Source: CAD feature listing. Evaluate the final solid. Frame: model axes, mm. A direction names the side the tool comes from. Give positions to 0.01 mm unless a question says otherwise; leave off trailing zeros. Order: outer loops, then holes, each group sorted by start corner. A loop starts at its lowest first (then second) coordinate and runs counter-clockwise, first axis right, second up.
from build123d import *

# Parameters (mm, degrees)
SKETCH1_R           = 11.5
BOSS_EXTRUDE1_DEPTH = 19
SKETCH2_R           = 0.6
BOSS_EXTRUDE4_DEPTH = 19
SKETCH3_R           = 3
BOSS_EXTRUDE5_DEPTH = 8.5
SKETCH4_R           = 1
CUT_EXTRUDE1_DEPTH  = 8.5


with BuildPart() as part:
    # Sketch1 → Boss-Extrude1 (new body)
    with BuildSketch(Plane.XY):
        Circle(SKETCH1_R)
    extrude(amount=BOSS_EXTRUDE1_DEPTH)

    # Sketch2 → Boss-Extrude4 (add)
    with BuildSketch(Plane(origin=(0, 0, 0), x_dir=(1, 0, 0), z_dir=(0, 1, 0))):
        with Locations((-2.2, -18.2)):
            Circle(SKETCH2_R)
        with Locations((-1.1, -18.2)):
            Circle(SKETCH2_R)
        with Locations((0, -18.2)):
            Circle(SKETCH2_R)
        with Locations((1.1, -18.2)):
            Circle(SKETCH2_R)
        with Locations((2.2, -18.2)):
            Circle(SKETCH2_R)
    extrude(amount=BOSS_EXTRUDE4_DEPTH)

    # Sketch3 → Boss-Extrude5 (add)
    with BuildSketch(Plane(origin=(0, 0, 0), x_dir=(-1, 0, 0), z_dir=(0, 0, -1))):
        Circle(SKETCH3_R)
    extrude(amount=BOSS_EXTRUDE5_DEPTH)

    # Sketch4 → Cut-Extrude1 (cut)
    with BuildSketch(Plane(origin=(0, 0, 0), x_dir=(-1, 0, 0), z_dir=(0, 0, -1))):
        with Locations((0, -8.5)):
            Circle(SKETCH4_R)
        with Locations((0, 8.5)):
            Circle(SKETCH4_R)
    extrude(amount=-CUT_EXTRUDE1_DEPTH, mode=Mode.SUBTRACT)


solid = part.part
1) Pull-direction query (Y, two-part tool) for faces 1 (the face through (0, 19, 18)), 2 (the face through (0, -8, 8.5)), 3 (the face through (2.4, -2.4, 0)); classes: +Y half, -Y half, draft (parallel to the pull), parting line (faces both ways), or undercut.
Checks:
face 1: +Y half
face 2: undercut
face 3: draft
2) First-contact query: pin 1 Ø8 at (y, z) = (11.5, 9) entering from +X; pin 2 Ø0.6 at (x, y) = (0.5, 8.5) entering from -Z; pin 3 Ø1 at (x, y) = (-5, 15) entering from -Z; pin 4 Ø8 at (x, z) = (8.5, -1) entering from +Y. Flat tips, straight axial feed; report the tip coordinate or a pass-through.
Checks:
pin 1: stops at x = 8.72
pin 2: stops at z = 8.5
pin 3: passes through
pin 4: stops at y = 10.53
3) Section query D-D on y = 0. Output: boundary loops of the cut face in (x, z).
Checks:
outline: (-11.5, 0) - (-3, 0) - (-3, -8.5) - (3, -8.5) - (3, 0) - (11.5, 0) - (11.5, 19) - (-11.5, 19) - close
4) Section query A-A on y = 17. Output: boundary loops of the cut face in (x, z).
Checks:
outline: (-1.65, 17.96) arc R0.6 ccw to (-0.55, 17.96) arc R0.6 ccw to (0.55, 17.96) arc R0.6 ccw to (1.65, 17.96) arc R0.6 ccw (long way) to (1.65, 18.44) arc R0.6 ccw to (0.55, 18.44) arc R0.6 ccw to (-0.55, 18.44) arc R0.6 ccw to (-1.65, 18.44) arc R0.6 ccw (long way) to start
5) Ray query, L1, parallel to Y at x = 0, z = 5.75; L2, parallel to Z at x = -4.25, y = 0; L3, parallel to X at y = -3.5, z = 8.25. Return the intervals inside material, ascending.
Checks:
L1: y = -11.5 to -9.5, -7.5 to 7.5, 9.5 to 11.5
L2: z = 0 to 19
L3: x = -10.95 to 10.95
6) Reachability of faces 4 (the face through (0, 0, -8.5)), 5 (the face through (0, 9, 8.5)) from +Z, -Z, +X, -X, +Y, -Y: full face, straight path, thin tool, end or side. Return the list, or none.
Checks:
face 4: -Z, +X, -X, +Y, -Y
face 5: -Z
7) Section query B-B on x = 0. Output: boundary loops of the cut face in (y, z).
Checks:
outline: (-11.5, 0) - (-9.5, 0) - (-9.5, 8.5) - (-7.5, 8.5) - (-7.5, 0) - (-3, 0) - (-3, -8.5) - (3, -8.5) - (3, 0) - (7.5, 0) - (7.5, 8.5) - (9.5, 8.5) - (9.5, 0) - (11.5, 0) - (11.5, 17.6) - (19, 17.6) - (19, 18.8) - (11.5, 18.8) - (11.5, 19) - (-11.5, 19) - close
8) Section query C-C on z = 11. Output: boundary loops of the cut face in (x, y), and give its area (3 significant figures).
Checks:
outline: circle Ø23 at (0, 0)
area: 415 mm2
